```python
from build123d import *

# Parameters (mm, degrees)
F0_W           = 20
F0_H           = 1.8
F1_DEPTH       = 45
F2_SIZE        = 2.5
F3_SIZE        = 2.5
F5_D           = 2
F5_DEPTH       = 15
F5_CSINK_D     = 6
F5_CSINK_ANGLE = 90


with BuildPart() as f1:
    # F0 (on Top) → F1 (new body)
    with BuildSketch(Plane.XY):
        Polygon((12, 3.40756), (-12, 3.40756), (-12, 1.60756), (-10, 1.60756), (10, 1.60756), (12, 1.60756), align=None)
        with Locations((0, 0.70756)):
            Rectangle(F0_W, F0_H)
    extrude(amount=F1_DEPTH)

    # F2
    f2_edges = [f1.edges().sort_by_distance(p)[0] for p in [
        (12, 2.50756, 0),
    ]]
    chamfer(f2_edges, length=F2_SIZE)

    # F3
    f3_edges = [f1.edges().sort_by_distance(p)[0] for p in [
        (-12, 2.50756, 0),
    ]]
    chamfer(f3_edges, length=F3_SIZE)

    # F5
    with Locations(Plane(origin=(0, 3.40756, 0), x_dir=(-1, 0, 0), z_dir=(0, 1, 0))):
        with Locations((0, 37), (0, 8)):
            CounterSinkHole(F5_D / 2, F5_CSINK_D / 2, depth=F5_DEPTH, counter_sink_angle=F5_CSINK_ANGLE)


solid = f1.part
```
Source: CAD feature listing. Evaluate the final solid. Frame: model axes, mm. A direction names the side the tool comes from. Round coordinates to 2 decimals unless told otherwise and drop trailing zeros. Write each loop counter-clockwise with the first axis right and the second up, starting at its lowest first coordinate (ties: lowest second). Pieces come first, ordered by that corner, then holes. Notation, with made-up numbers: M -7.5,74.25 L 49.5,74.25 A22 ccw 49.5,102.25 Z; hole C -24,25.25 d9. An arc over 180 degrees is marked long. Use CSV: the item, a comma, the result in double quotes. Start each with the question number.
Q1. Access query for faces 1 (the face through (0, 2, 45)), 2 (the face through (10, 1, 22)), 3 (the face through (-10, 1, 22)). Directions: +Z, -Z, +X, -X, +Y, -Y. A direction counts if a zero-diameter tool reaches every point of the face in a straight line with its end or side. Return the directions, or none.
Q2. Line query: line 1 (Z direction, x = 0, y = 1); line 2 (X direction, y = 0.55, z = 37); line 3 (X direction, y = 0.55, z = 32). Output: solid intervals per line, ascending. Write a range as from..to.
Q3. First-contact query: P1, Ø0.6, axis at x = -11, z = 29.5, coming from the -Y side; P2, Ø1.5, axis at y = 0.5, z = 31.5, coming from the +X side; P3, Ø1.8, axis at x = 0, z = 37, coming from the +Y side; P4, Ø1.4, axis at y = 0.5, z = 15.5, coming from the -X side. Flat tips, straight axial feed; report the tip coordinate or a pass-through.
Q4. Cut plane C-C on y = 0.4. Output: boundary loops of the cut face in (x, z), plus the area to 3 significant figures.
Q5. Cut plane D-D on z = 23.5. Output: boundary loops of the cut face in (x, y), plus the area to 3 significant figures.
Q6. Pull-direction query (Z, two-part tool) for faces 4 (the face through (11, 1.608, 22)), 5 (the face through (0, 1, 9)), 6 (the face through (0, 2, 0)); classes: +Z half, -Z half, draft (parallel to the pull), parting line (faces both ways), or undercut.
Q7. Cut plane B-B on z = 37. Output: boundary loops of the cut face in (x, y).
Q8. Cut plane A-A on x = 0. Output: boundary loops of the cut face in (y, z), plus the area to 3 significant figures.
Results found:
1,face 1,"+Z, +X, -X, +Y, -Y"
1,face 2,"+Z, -Z, +X, -Y"
1,face 3,"+Z, -Z, -X, -Y"
2,line 1,"0..7, 9..36, 38..45"
2,line 2,"-10..-1, 1..10"
2,line 3,"-10..10"
3,P1,"y = 1.61"
3,P2,"x = 10"
3,P3,"through"
3,P4,"x = -10"
4,outline,"M -10,0.5 L -9.5,0 L 9.5,0 L 10,0.5 L 10,45 L -10,45 Z; hole C 0,8 d2; hole C 0,37 d2"
4,area,"893 mm^2"
5,outline,"M -12,1.61 L -10,1.61 L -10,-0.19 L 10,-0.19 L 10,1.61 L 12,1.61 L 12,3.41 L -12,3.41 Z"
5,area,"79.2 mm^2"
6,face 4,"draft"
6,face 5,"undercut"
6,face 6,"-Z half"
7,outline,"M -12,1.61 L -10,1.61 L -10,-0.19 L -1,-0.19 L -1,1.41 L -3,3.41 L -12,3.41 Z; M 1,-0.19 L 10,-0.19 L 10,1.61 L 12,1.61 L 12,3.41 L 3,3.41 L 1,1.41 Z"
8,outline,"M -0.19,0 L 3.41,0 L 3.41,5 L 1.41,7 L -0.19,7 Z; M -0.19,9 L 1.41,9 L 3.41,11 L 3.41,34 L 1.41,36 L -0.19,36 Z; M -0.19,38 L 1.41,38 L 3.41,40 L 3.41,45 L -0.19,45 Z"
8,area,"140 mm^2"
